Build history of the part. All positions in model axes, mm. Face numbers are marked on the shaded views. A direction names the side the tool comes from. Give positions to 0.01 mm unless a question says otherwise; leave off trailing zeros. Write each loop counter-clockwise with the first axis right and the second up, starting at its lowest first coordinate (ties: lowest second). Pieces come first, ordered by that corner, then holes.
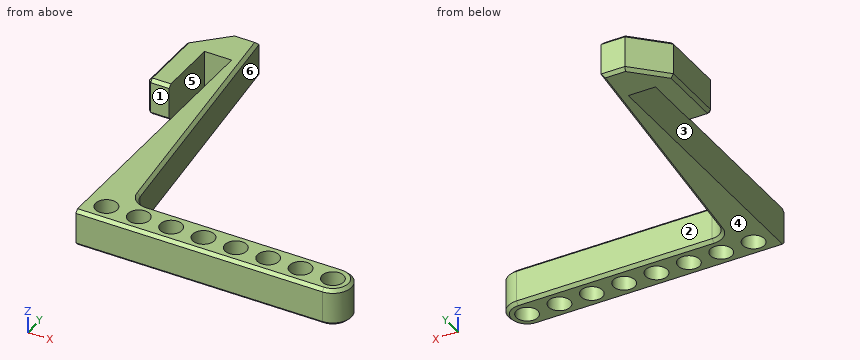
from build123d import *

# Parameters (mm, degrees)
F0_R     = 3.5
F1_DEPTH = 12
F3_DEPTH = 25
F4_R     = 5
F5_W     = 12
F5_H     = 12
F6_DEPTH = 15.8
F7_W     = 7
F7_H     = 12
F8_DEPTH = 20
F9_SIZE  = 10
F10_SIZE = 1


with BuildPart() as f1:
    # F0 (on Top) → F1 (new body)
    with BuildSketch(Plane.XY):
        with BuildLine():
            Line((12, 100), (0, 100))
            Line((0, 100), (0, 0))
            Line((0, 0), (80, 0))
            ThreePointArc((80, 0), (86, 6), (80, 12))
            Line((80, 12), (12, 12))
            Line((12, 12), (12, 100))
        make_face()
        with Locations((6.5, 6)):
            Circle(F0_R, mode=Mode.SUBTRACT)
        with Locations((17, 6)):
            Circle(F0_R, mode=Mode.SUBTRACT)
        with Locations((27.5, 6)):
            Circle(F0_R, mode=Mode.SUBTRACT)
        with Locations((38, 6)):
            Circle(F0_R, mode=Mode.SUBTRACT)
        with Locations((48.5, 6)):
            Circle(F0_R, mode=Mode.SUBTRACT)
        with Locations((59, 6)):
            Circle(F0_R, mode=Mode.SUBTRACT)
        with Locations((69.5, 6)):
            Circle(F0_R, mode=Mode.SUBTRACT)
        with Locations((80, 6)):
            Circle(F0_R, mode=Mode.SUBTRACT)
    extrude(amount=F1_DEPTH)

    # F2 (on face) → F3 (cut)
    with BuildSketch(Plane.XY.offset(12)):
        Polygon((2, 100), (12, 12), (12, 100), align=None)
    extrude(amount=-F3_DEPTH, mode=Mode.SUBTRACT)

    # F4
    f4_edges = [f1.edges().sort_by_distance(p)[0] for p in [
        (12, 12, 6),
    ]]
    fillet(f4_edges, radius=F4_R)

    # F5 (on face) → F6 (join)
    with BuildSketch(Plane(origin=(0, 0, 0), x_dir=(0, -1, 0), z_dir=(-1, 0, 0))):
        with Locations((-94, 6)):
            Rectangle(F5_W, F5_H)
    extrude(amount=F6_DEPTH)

    # F7 (on face) → F8 (join)
    with BuildSketch(Plane.XZ.offset(-88)):
        with Locations((-12.3, 6)):
            Rectangle(F7_W, F7_H)
    extrude(amount=F8_DEPTH)

    # F9
    f9_edges = [f1.edges().sort_by_distance(p)[0] for p in [
        (-15.8, 100, 6),
    ]]
    chamfer(f9_edges, length=F9_SIZE)

    # F10
    f10_edges = [f1.edges().sort_by_distance(p)[0] for p in [
        (6.747986, 58.217726, 12),
        (6.747986, 58.217726, 0),
        (-1.9, 100, 12),
        (-10.8, 95, 12),
        (-15.8, 79, 12),
        (-1.9, 100, 0),
        (-10.8, 95, 0),
        (-15.8, 79, 0),
        (-15.8, 68, 6),
        (-12.3, 68, 12),
        (-12.3, 68, 0),
    ]]
    chamfer(f10_edges, length=F10_SIZE)


solid = f1.part
1. Saw through at B-B on z = 3.25. Count the separate pieces of the cut face and the enclosed holes in it, plus the area to 3 significant figures.
2. Saw through at A-A on x = 69.5. Give the cut face in (y, z).
3. Drill centre lines: line 1 along Y through (x, z) = (38, 3.5); line 2 along Y through (x, z) = (42, 4); line 3 along X through (y, z) = (80, 10.75). Where is each one in solid material? Low to high.
4. Mould opens along X. For the marked faces 4, 5 and 6 say: pulls with the +X half, pulls with the -X half, needs draft (parallel to the pull), parting line crosses it, or undercut.
5. Drop flat-ended pins along their axis: pin 1 (4.5 mm diameter, centred on x = -3, z = 9, fed in from -Y); pin 2 (6.5 mm diameter, centred on x = -11.5, z = 7, fed in from -Y); pin 3 (1.5 mm diameter, centred on y = 86, z = 5, fed in from +X). Give the stop position or say it passes through.
6. 3-axis set-ups, long thin cutter, end or side, ignore diameter. For the marked faces 1, 2 and 3: which of +Z, -Z, +X, -X, +Y, -Y reach the whole face in a straight line?
7. Saw through at C-C on x = 32.5. Give the cut face in (y, z), plus the area to 3 significant figures.
Outcome:
1. separate pieces: 1
1. enclosed holes: 8
1. area: 1,610 mm2
2. outline: (0, 1) - (1, 0) - (2.5, 0) - (2.5, 12) - (1, 12) - (0, 11) - close; (9.5, 0) - (11, 0) - (12, 1) - (12, 11) - (11, 12) - (9.5, 12) - close
3. line 1: y = 0 to 2.5, 9.5 to 12
3. line 2: y = 0 to 12
3. line 3: x = -15.8 to -8.8, 0 to 4.27
4. face 4: needs draft
4. face 5: undercut
4. face 6: pulls with the +X half
5. pin 1: stops at y = 88
5. pin 2: stops at y = 68
5. pin 3: stops at x = 3.68
6. face 1: +Z, -Z, -X, -Y
6. face 2: +Z, -Z, +X, +Y
6. face 3: +Z, -Z, -Y
7. outline: (0, 1) - (1, 0) - (11, 0) - (12, 1) - (12, 11) - (11, 12) - (1, 12) - (0, 11) - close
7. area: 142 mm2
